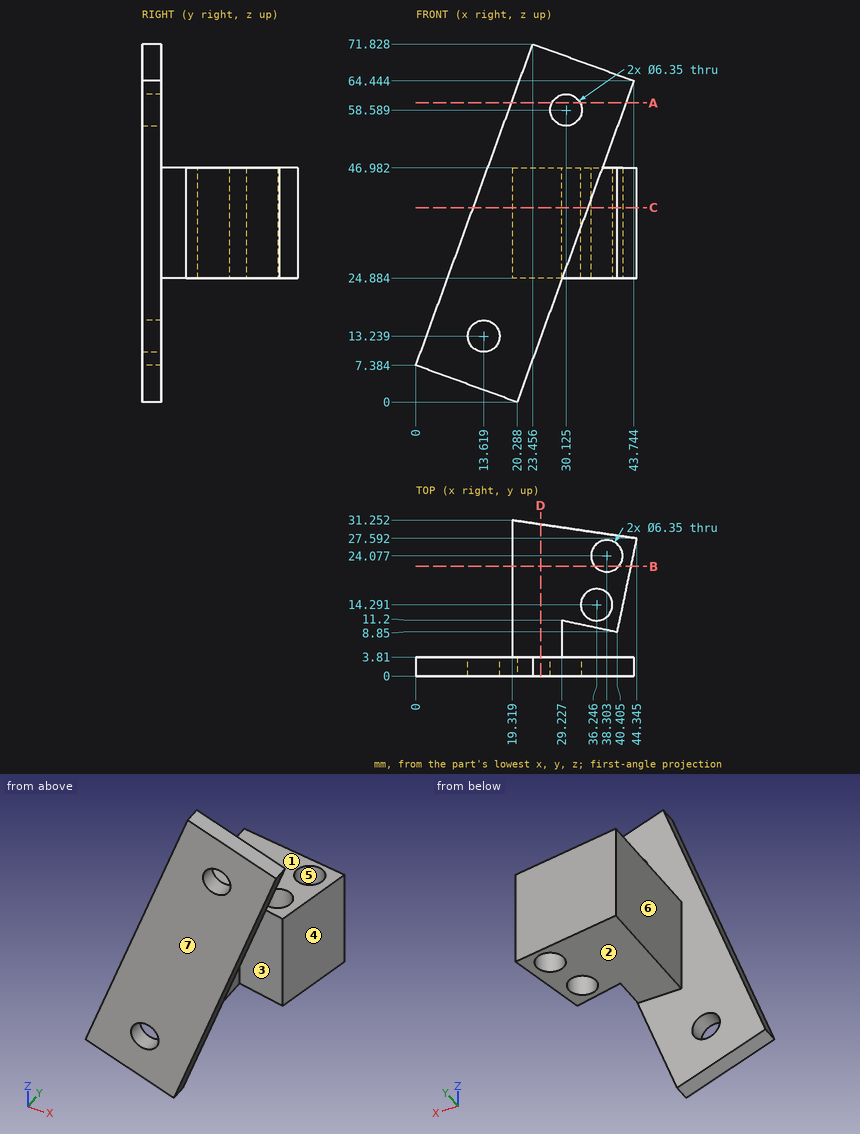
Study the drawing (mm; zero at the part's minimum x, y, z) and answer. A direction names the side the tool comes from. Give positions to 0.01 mm unless a question says otherwise; leave off trailing zeros. Order: outer loops, then holes, each group sorted by start corner. A loop starts at its lowest first (then second) coordinate and runs counter-clockwise, first axis right, second up.
1. Section C-C, the plane z = 39 is taken. Give the number of separate pieces and of enclosed holes in the cut face, and give its area (3 significant figures).
Result sheet:
separate pieces: 1
enclosed holes: 2
area: 539 mm2
2. For the marked faces 1, 2 and 3, determine the directions among +Z, -Z, +X, -X, +Y, -Y from which every point of the face is accessible in a straight line to the end or side of a thin tool.
Result sheet:
face 1: +Z, +X, -X, +Y
face 2: -Z, +X, -X, +Y
face 3: +Z, -Z
3. Section A-A, the plane z = 60 is taken. Determine the outline of the cut face in (x, y).
Result sheet:
outline: (19.15, 0) - (27.28, 0) - (27.28, 3.81) - (19.15, 3.81) - close; (32.97, 0) - (42.13, 0) - (42.13, 3.81) - (32.97, 3.81) - close
4. Straight lines are drawn through the part: L1, parallel to Y at x = 27, z = 63; L2, parallel to Z at x = 27.5, y = 13.5; L3, parallel to Y at x = 19.5, z = 39 (1 decimal). For each, find the intervals that lie inside material, in ascending order.
Result sheet:
L1: y = 0 to 3.81
L2: z = 24.88 to 46.98
L3: y = 0 to 31.2
5. The mould has two halves that part along X. Classify the marked faces 4, 5, 6 and 7: released by +X, released by -X, zero draft, split by the parting line, or undercut.
Result sheet:
face 4: released by +X
face 5: undercut
face 6: released by -X
face 7: zero draft
6. Section D-D, the plane x = 25 is taken. Determine the outline of the cut face in (y, z).
Result sheet:
outline: (0, 12.95) - (3.81, 12.95) - (3.81, 24.88) - (30.42, 24.88) - (30.42, 46.98) - (3.81, 46.98) - (3.81, 71.27) - (0, 71.27) - close
7. Each of these flat-tipped pins is pushed along its axis until it touches: P1, Ø5.5, axis at x = 13.62, z = 13.24, coming from the +Y side; P2, Ø10, axis at x = 36.5, y = 26.5, coming from the +Z side; P3, Ø10, axis at x = 27.5, z = 61, coming from the +Y side; P4, Ø5, axis at y = 7, z = 36, coming from the +X side. Where does it stop, or does it pass through?
Result sheet:
P1: passes through
P2: stops at z = 46.98
P3: stops at y = 3.81
P4: stops at x = 40.54
8. Section B-B, the plane y = 22 is taken. Determine the outline of the cut face in (x, z) (1 decimal).
Result sheet:
outline: (19.3, 24.9) - (35.9, 24.9) - (35.9, 47) - (19.3, 47) - close; (40.7, 24.9) - (43.2, 24.9) - (43.2, 47) - (40.7, 47) - close
